Job drawing, mm, ordinate dimensions from the low corner. One solid piece. A direction names the side the tool comes from. Round coordinates to 2 decimals unless told otherwise and drop trailing zeros. Write each loop counter-clockwise with the first axis right and the second up, starting at its lowest first coordinate (ties: lowest second). Pieces come first, ordered by that corner, then holes. Notation, with made-up numbers: M 87,10 L 112,10 A29 ccw 112,43 Z; hole C -19.5,45.25 d7. An arc over 180 degrees is marked long. One line per item, written item: value. Start each with the question number.
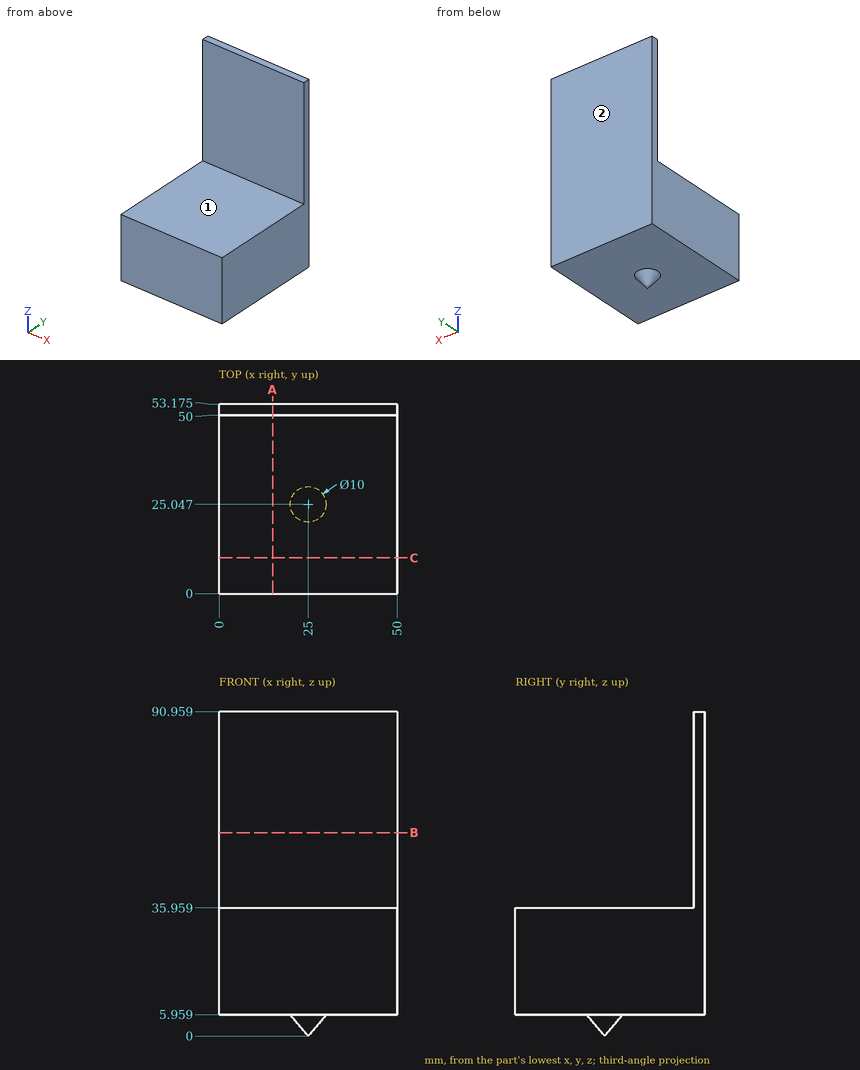
Item 1: Which spindle directions (+Z, -Z, +X, -X, +Y, -Y) get a long thin tool onto all of the face, cutting with end or side? Do the marked faces 1 and 2. Say none if no direction does.
Item 2: Cut at A-A, the plane x = 15. Write the cut outline in (y, z) (1 decimal), plus the area to 3 significant figures.
Item 3: Cut at B-B, the plane z = 57. Write the cut outline in (x, y) (1 decimal).
Item 4: Drill centre lines: line 1 (Z direction, x = 23.5, y = 7.5); line 2 (Y direction, x = 5.5, z = 46.5) (1 decimal); line 3 (Z direction, x = 25, y = 25.5). Where is each one in solid material? Low to high.
Item 5: Drop flat-ended pins along their axis: pin 1 (25 mm diameter, centred on x = 24, z = 66, fed in from -Y); pin 2 (12 mm diameter, centred on x = 24.5, y = 26.5, fed in from +Z); pin 3 (1 mm diameter, centred on x = 27, y = 14, fed in from -Z). Give the stop position or say it passes through.
Item 6: Cut at C-C, the plane y = 10. Write the cut outline in (x, z).
Computed values:
1. face 1: +Z, +X, -X, -Y
1. face 2: +Z, -Z, +X, -X, +Y
2. outline: M 0,6 L 53.2,6 L 53.2,91 L 50,91 L 50,36 L 0,36 Z
2. area: 1,770 mm2
3. outline: M 0,50 L 50,50 L 50,53.2 L 0,53.2 Z
4. line 1: z = 5.96 to 35.96
4. line 2: y = 50 to 53.2
4. line 3: z = 0.54 to 35.96
5. pin 1: stops at y = 50
5. pin 2: stops at z = 35.96
5. pin 3: stops at z = 5.96
6. outline: M 0,5.96 L 50,5.96 L 50,35.96 L 0,35.96 Z
